from build123d import *

# Parameters (mm, degrees)
SKETCH_2_R          = 1
CUT_EXTRUDE_1_DEPTH = 4
SKETCH_3_R          = 1
CUT_EXTRUDE_2_DEPTH = 3


with BuildPart() as part:
    # 草图1 → 旋转1 (revolve)
    with BuildSketch(Plane.XY, mode=Mode.PRIVATE) as revolve_1_sk:
        Polygon((0, 19.290656643), (0, 0), (0, -4.509343357), (1, -4.509343357), (1, -2.709343357), (9.5, -2.709343357), (11.5, -0.709343357), (11.5, 0.290656643), (11, 0.290656643), (11, 0.790656643), (11.5, 0.790656643), (11.5, 1.790656643), (9.5, 1.790656643), (9.5, 2.290656643), (11.5, 2.290656643), (11.5, 11.790656643), (7.5, 15.790656643), (1, 15.790656643), (1, 19.290656643), align=None)
        Polygon((2, 14.790656643), (7.085786438, 14.790656643), (10.5, 11.376443081), (10.5, 10.251588649), (1, 10.251588649), (1, 13.790656643), (2, 13.790656643), align=None, mode=Mode.SUBTRACT)
    revolve(revolve_1_sk.sketch.rotate(Axis((0, 19.290656643, 0), (0, -1, 0)), 90), axis=Axis((0, 19.290656643, 0), (0, -1, 0)))

    # 草图2 → 切除-拉伸1 (cut)
    with BuildSketch(Plane(origin=(0, 15.790656643, 0), x_dir=(1, 0, 0), z_dir=(0, 1, 0))):
        with Locations(Location((0, -4.5, 0), (0, 0, 270))):
            Circle(SKETCH_2_R)
        with Locations(Location((-4.5, 0, 0), (0, 0, 270))):
            Circle(SKETCH_2_R)
        with Locations(Location((0, 4.5, 0), (0, 0, 270))):
            Circle(SKETCH_2_R)
        with Locations(Location((4.5, 0, 0), (0, 0, 270))):
            Circle(SKETCH_2_R)
        with BuildLine():
            Line((-3, 9), (-3, 16.559368986))
            Line((-3, 16.559368986), (3, 16.559368986))
            Line((3, 16.559368986), (3, 9))
            ThreePointArc((3, 9), (0, 6), (-3, 9))
        make_face()
        with BuildLine():
            Line((15.840834213, 5.681608282), (12.840834213, 10.877760704))
            Line((12.840834213, 10.877760704), (6.294228634, 7.098076211))
            ThreePointArc((6.294228634, 7.098076211), (5.196152423, 3), (9.294228634, 1.901923789))
            Line((9.294228634, 1.901923789), (15.840834213, 5.681608282))
        make_face()
        with BuildLine():
            Line((12.840834213, -10.877760704), (15.840834213, -5.681608282))
            Line((15.840834213, -5.681608282), (9.294228634, -1.901923789))
            ThreePointArc((9.294228634, -1.901923789), (5.196152423, -3), (6.294228634, -7.098076211))
            Line((6.294228634, -7.098076211), (12.840834213, -10.877760704))
        make_face()
        with BuildLine():
            Line((-3, -16.559368986), (3, -16.559368986))
            Line((3, -16.559368986), (3, -9))
            ThreePointArc((3, -9), (0, -6), (-3, -9))
            Line((-3, -9), (-3, -16.559368986))
        make_face()
        with BuildLine():
            Line((-15.840834213, -5.681608282), (-12.840834213, -10.877760704))
            Line((-12.840834213, -10.877760704), (-6.294228634, -7.098076211))
            ThreePointArc((-6.294228634, -7.098076211), (-5.196152423, -3), (-9.294228634, -1.901923789))
            Line((-9.294228634, -1.901923789), (-15.840834213, -5.681608282))
        make_face()
        with BuildLine():
            Line((-12.840834213, 10.877760704), (-15.840834213, 5.681608282))
            Line((-15.840834213, 5.681608282), (-9.294228634, 1.901923789))
            ThreePointArc((-9.294228634, 1.901923789), (-5.196152423, 3), (-6.294228634, 7.098076211))
            Line((-6.294228634, 7.098076211), (-12.840834213, 10.877760704))
        make_face()
    extrude(amount=-CUT_EXTRUDE_1_DEPTH, mode=Mode.SUBTRACT)

    # 草图3 → 切除-拉伸2 (cut)
    with BuildSketch(Plane.XZ.offset(2.709343357)):
        with Locations(Location((0, 6, 0), (0, 0, 270))):
            Circle(SKETCH_3_R)
        with Locations(Location((0, -6, 0), (0, 0, 270))):
            Circle(SKETCH_3_R)
        with Locations(Location((-8, 0, 0), (0, 0, 270))):
            Circle(SKETCH_3_R)
        with Locations(Location((8, 0, 0), (0, 0, 270))):
            Circle(SKETCH_3_R)
    extrude(amount=-CUT_EXTRUDE_2_DEPTH, mode=Mode.SUBTRACT)


solid = part.part
Could you check a few things on this model? Use its own coordinates, in mm. A direction names the side the tool comes from. Coordinates: 2 decimals unless noted, no trailing zeros. Order: outer loops, then holes, each group sorted by start corner. A loop starts at its lowest first (then second) coordinate and runs counter-clockwise, first axis right, second up. Notation, with made-up numbers: (9, -26.75) -> (22, -26.75) arc R23 cw to (22, -14.75) -> close; hole circle Ø7 at (-2.5, 56). An arc over 180 degrees is marked (long way). One line per item, written item: value. Start each with the question number.
1) Imagine slicing it at A-A on x = 0.5. Count the separate pieces of the cut face and the enclosed holes in it, plus the area to 3 significant figures.
2) If I drill on L1, parallel to Y at x = 3.25, z = 0; L2, parallel to X at y = 15.3, z = 0; L3, parallel to X at y = -1.55, z = 0, over which ranges is the centre line in solid material (lowest first)? Write a range as [from, to].
3) I'm going to push flat-ended pins straight in: pin 1 (1 mm diameter, centred on x = 5.5, z = 3, fed in from +Y); pin 2 (0.6 mm diameter, centred on x = 1, z = 10.5, fed in from +Y); pin 3 (1.2 mm diameter, centred on x = 0, z = 4.5, fed in from -Y). Where does each tip first touch, or does it pass through?
4) We'd pull the mould along Z, two halves only. Please class faces 1 (the flat face through (2, -2.709, 0)), 2 (the flat face through (-10.015, 12.588, -2.318)), 3 (the cylindrical face through (-5.164, 15.248, 3.057)): +Z half, -Z half, draft (parallel to the pull), parting line (faces both ways), or undercut.
5) Which directions (+Z, -Z, +X, -X, +Y, -Y) give clear straight access to the entire face, cutting with the end or side of a thin tool? Please do faces 4 (the cylindrical face through (-3.2, 10.8, 10)), 5 (the flat face through (-3, 12.6, 9.8)), 6 (the flat face through (0, 0.291, 6)).
6) Imagine slicing it at C-C on y = 7. List the corners of the cut face in (x, z) for me.
Answer list:
1. separate pieces: 3
1. enclosed holes: 0
1. area: 312 mm2
2. L1: y = [-2.71, 10.25], [14.79, 15.79]
2. L2: x = [-7.99, -5.5], [-3.5, 3.5], [5.5, 7.99]
2. L3: x = [-10.66, -9], [-7, 7], [9, 10.66]
3. pin 1: stops at y = 15.79
3. pin 2: stops at y = 11.79
3. pin 3: stops at y = -2.71
4. face 1: draft
4. face 2: -Z half
4. face 3: undercut
5. face 4: none
5. face 5: +Z, +Y
5. face 6: -Y
6. outline: circle Ø23 at (0, 0)
